Verification items for the finished model (mm, model axes). Round coordinates to 2 decimals unless told otherwise and drop trailing zeros. Write each loop counter-clockwise with the first axis right and the second up, starting at its lowest first coordinate (ties: lowest second). Pieces come first, ordered by that corner, then holes. Notation, with made-up numbers: M 30,-5 L 59,-5 A11 ccw 59,6 Z; hole C 44,86 d8. An arc over 180 degrees is marked long. Use a Markdown table: item, result. Add a question column.
from build123d import *

# Parameters (mm, degrees)
EXTRUDE_1_DEPTH = 5


with BuildPart() as part:
    # Model → 凸台-拉伸1 (new body)
    with BuildSketch(Plane.XY):
        Polygon((67.236808621, 3.639203016), (69.436808621, 3.639203016), (69.436808621, 2.639203016), (99.083381953, 2.639203016), (99.083381953, 3.639203016), (101.283381953, 3.639203016), (101.283381953, 2.639203016), (131.03665326, 2.639203016), (131.03665326, 3.62337358), (133.236025848, 3.639203016), (133.236025848, 2.639203016), (176.136025848, 2.639203016), (176.136025848, 3.639203016), (178.336025848, 3.639203016), (178.336025848, 8.639203016), (50.336025848, 8.639203016), (3.336025848, 8.639203016), (3.336025848, 3.639203016), (7.736025848, 3.639203016), (7.736025848, 2.639203016), (21.308226604, 2.639203016), (21.308226604, 3.639203016), (25.708226604, 3.639203016), (25.708226604, 2.639203016), (67.236808621, 2.639203016), align=None)
    extrude(amount=EXTRUDE_1_DEPTH)


solid = part.part
1. Cross-section at A-A on z = 2.55. Enter the section's corners in (x, y).
2. Release check for a two-part mould opening along X. For faces 1 (the flat face through (6, 3.639, 2)), 2 (the flat face through (23, 3.639, 2)), 3 (the flat face through (178.336, 6, 2)) record: +X half, -X half, draft (parallel to the pull), parting line (faces both ways), or undercut.
3. Depth check by flat-ended pin: pin 1 Ø1.3 at (x, z) = (6.5, 2) entering from -Y; pin 2 Ø1.1 at (y, z) = (3, 2) entering from -X; pin 3 Ø0.5 at (y, z) = (3, 2.5) entering from +X. Enter the tip coordinate at first touch or a pass-through.
4. Scan line: line 1 along Y through (x, z) = (132, 0.4). Record every from-to range of solid material in increasing order. Write a range as from..to.
Answer:
| question | item | result |
|---|---|---|
| 1 | outline | M 3.34,3.64 L 7.74,3.64 L 7.74,2.64 L 21.31,2.64 L 21.31,3.64 L 25.71,3.64 L 25.71,2.64 L 67.24,2.64 L 67.24,3.64 L 69.44,3.64 L 69.44,2.64 L 99.08,2.64 L 99.08,3.64 L 101.28,3.64 L 101.28,2.64 L 131.04,2.64 L 131.04,3.62 L 133.24,3.64 L 133.24,2.64 L 176.14,2.64 L 176.14,3.64 L 178.34,3.64 L 178.34,8.64 L 3.34,8.64 Z |
| 2 | face 1 | draft |
| 2 | face 2 | undercut |
| 2 | face 3 | +X half |
| 3 | pin 1 | stops at y = 3.64 |
| 3 | pin 2 | stops at x = 7.74 |
| 3 | pin 3 | stops at x = 176.14 |
| 4 | line 1 | y = 3.63..8.64 |
